Autodesk Inventor part; units mm, degrees
sketch "Sketch1" plane through (0, 0, 0) normal (1, 0, 0) x (0, 1, 0)
  circle A0 centre (30.5, -5.5) radius 3.5
  line L0 (11, 15) -> (5, 15)
  line L1 (5, -15) -> (11, -15)
  line L2 (0, -21) -> (5, -21)
  line L3 (5, -21) -> (5, -15)
  line L4 (0, 21) -> (5, 21)
  line L5 (5, 21) -> (5, 15)
  line L6 (-7.7302, 0) -> (46.3815, 0)
  line L7 (0, 29.4) -> (0, -29.4)
  line L8 (0, 21) -> (0, -21)
  line L9 (11, -15) -> (23.6512, -15)
  line L10 (11, 15) -> (23.6512, 15)
  arc A1 (23.6512, -15) -> (23.6512, 15) centre (23.6512, 0) ccw
  circle A2 centre (11, 0) radius 5
  point P0 (2.5, -21)
  dimension "d7" = 7
  dimension "d45" = 21
  dimension "d64" = 5
  dimension "d65" = 21
  dimension "d66" = 5
  dimension "d67" = 15
  dimension "d69" = 5.5
  dimension "d73" = 0
  dimension "d74" = 30.5
  dimension "d75" = 10
  dimension "d76" = 0
  dimension "d77" = 11
  dimension "d78" = 15
  dimension "d79" = 15
  dimension "d80" = 23.6512
extrude "Extrusion1" add sketch "Sketch1" along normal blind 10 contours L10 A1 L6 A2 L7 L4 L5 L0 | A1 L9 L1 L3 L2 L7 L6 A2
sketch "Sketch4" plane through (10, 0, 0) normal (1, 0, 0) x (0, 0, -1)
  circle A0 centre (0, 11) radius 9.5
  line L0 (-29.4, 0) -> (29.4, 0)
  line L1 (0, -7.7302) -> (0, 46.3815)
  point P0 (0, 0)
  dimension "d56" = 19
  dimension "d58" = 11
  dimension "d59" = 0
extrude "Extrusion2" cut sketch "Sketch4" along normal blind 6 from surface at -10
sketch "Sketch6" plane through (0, 5, -15) normal (0, 1, 0) x (1, 0, 0)
  circle A0 centre (5, 3) radius 1.5
  line L0 (12, -15) -> (-2, -15)
  circle A1 centre (5, -33) radius 1.5
  line L1 (0, -30) -> (0, -36)
  line L2 (0, 6) -> (0, 0)
  point P0 (0, -15)
  point P1 (0, -33)
  point P2 (0, 3)
  dimension "d81" = 3
  dimension "d82" = 18
  dimension "d83" = 3
  dimension "d84" = 18
  dimension "d85" = 5
  dimension "d86" = 5
extrude "Extrusion3" cut sketch "Sketch6" against normal blind 5
sketch "Sketch7" plane through (0, 0, 0) normal (-1, 0, 0) x (0, 0, 1)
  circle A0 centre (-5.5, 30.5) radius 5
  line L0 (21, 0) -> (-21, 0)
  line L1 (0, -7.7302) -> (0, 46.3815)
  point P0 (0, 0)
  dimension "d89" = 10
  dimension "d90" = 30.5
  dimension "d91" = 5.5
extrude "Extrusion4" cut sketch "Sketch7" against normal blind 4
properties part number "support_arriere_droite"
Input: part model. Units: mm. Frame: model coordinates. A direction names the side the tool comes from. Coordinates: 2 decimals unless noted, no trailing zeros. Order: outer loops, then holes, each group sorted by start corner. A loop starts at its lowest first (then second) coordinate and runs counter-clockwise, first axis right, second up. Notation, with made-up numbers: M 36,51 L 58,51 A21 ccw 58,57 Z; hole C -31,26.5 d2. An arc over 180 degrees is marked long. Answer in a Markdown table with one row per item.
(1) Draft query along Z for faces 4 (the flat face through (5, 2, -21)), 5 (the cylindrical face through (7.97, 15.77, -1.5)), 6 (the flat face through (6, 7, -4)), 7 (the flat face through (10, 19, 0)). Return one class per face: pulls with the +Z half, pulls with the -Z half, needs draft (parallel to the pull), parting line crosses it, or undercut.
Numbers:
| item | result |
|---|---|
| face 4 | pulls with the -Z half |
| face 5 | undercut |
| face 6 | undercut |
| face 7 | needs draft |
(2) Access query for faces 1 (the flat face through (3.8, 5, 19.4)), 2 (the flat face through (4, 29, -9)), 3 (the flat face through (5, 14, -15)). Directions: +Z, -Z, +X, -X, +Y, -Y. A direction counts if a zero-diameter tool reaches every point of the face in a straight line with its end or side. Return the directions, or none.
Numbers:
| item | result |
|---|---|
| face 1 | +Z, +X, -X, +Y |
| face 2 | -X |
| face 3 | -Z, +X, -X, +Y |
(3) Section query C-C, the plane y = 11. Output: boundary loops of the cut face in (x, z), plus the area to 3 significant figures.
Numbers:
| item | result |
|---|---|
| outline | M 0,-15 L 10,-15 L 10,-5 L 6,-5 L 6,-9.5 L 0,-9.5 Z; M 0,9.5 L 6,9.5 L 6,5 L 10,5 L 10,15 L 0,15 Z |
| area | 146 mm^2 |
(4) Contact query for flat-ended pins moving along their axis: pin 1 Ø3 at (x, y) = (3.5, 16) entering from +Z; pin 2 Ø5.5 at (y, z) = (10.5, 3) entering from -X; pin 3 Ø1.8 at (x, z) = (7, -18.5) entering from +Y. Output: stop coordinate, or through.
Numbers:
| item | result |
|---|---|
| pin 1 | stops at z = 15 |
| pin 2 | stops at x = 6 |
| pin 3 | stops at y = 5 |
(5) Section query D-D, the plane x = 7.25. Output: boundary loops of the cut face in (y, z).
Numbers:
| item | result |
|---|---|
| outline | M 0,-21 L 5,-21 L 5,-15 L 23.65,-15 A15 ccw 23.65,15 L 5,15 L 5,21 L 0,21 Z; hole C 11,0 d10; hole C 30.5,-5.5 d7 |
(6) Section query B-B, the plane z = -18. Output: boundary loops of the cut face in (x, y).
Numbers:
| item | result |
|---|---|
| outline | M 0,0 L 3.5,0 L 3.5,5 L 0,5 Z; M 6.5,0 L 10,0 L 10,5 L 6.5,5 Z |
(7) Section query A-A, the plane x = 5. Output: boundary loops of the cut face in (y, z), plus the area to 3 significant figures.
Numbers:
| item | result |
|---|---|
| outline | M 0,-21 L 5,-21 L 5,-19.5 L 0,-19.5 Z; M 0,-16.5 L 5,-16.5 L 5,-15 L 23.65,-15 A15 ccw 23.65,15 L 5,15 L 5,16.5 L 0,16.5 Z; M 0,19.5 L 5,19.5 L 5,21 L 0,21 Z; hole C 11,0 d19; hole C 30.5,-5.5 d7 |
| area | 771 mm^2 |
(8) Material intervals for line 1 (X direction, y = 1, z = 18); line 2 (Y direction, x = 3, z = 0); line 3 (Y direction, x = 9.2, z = 0), sorted ascending. Write a range as [from, to].
Numbers:
| item | result |
|---|---|
| line 1 | x = [0, 3.5], [6.5, 10] |
| line 2 | y = [0, 1.5], [20.5, 38.65] |
| line 3 | y = [0, 6], [16, 38.65] |
